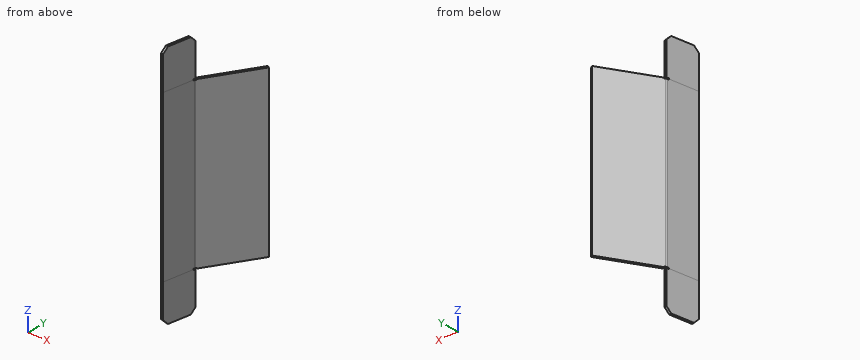
```python
from build123d import *

# Parameters (mm, degrees)
BOSS_EXTRUDE1_DEPTH      = 109.5375
BOSS_EXTRUDE1_DEPTH_BACK = 109.5375
SKETCH2_W                = 50.8
SKETCH2_H                = 42.97785953
BOSS_EXTRUDE2_DEPTH      = 3.175
CHAMFER1_SIZE            = 6.35
CONVERT_SOLID1_START     = -110.33125
CONVERT_SOLID1_DEPTH     = 220.6625
CONVERT_SOLID1_2_DEPTH   = 1.5875
CONVERT_SOLID1_START_2   = 108.74375
CONVERT_SOLID1_3_DEPTH   = 1.5875
CONVERT_SOLID1_START_3   = -108.74375
CONVERT_SOLID1_4_DEPTH   = 217.4875


# Read off the part's stored shape, not the designer's step: Convert-Solid1
with BuildPart() as part:
    # Sketch1 → Boss-Extrude1 (new, two sides: drawn at the far end of the back side and taken through both)
    with BuildSketch(Plane.XY.offset(-BOSS_EXTRUDE1_DEPTH_BACK)):
        Polygon((640.29736406, 709.2417051), (646.924037824, 751.080876614), (687.413907929, 818.467336674), (684.69240175, 820.102582562), (643.884672043, 752.187115289), (637.161453578, 709.738384527), align=None)
    extrude(amount=BOSS_EXTRUDE1_DEPTH + BOSS_EXTRUDE1_DEPTH_BACK)

    # Sketch2 → Boss-Extrude2 (add)
    with BuildSketch(Plane(origin=(511.908391779, -81.078324129, 0), x_dir=(0, 0, 1), z_dir=(-0.9876883405951397, 0.1564344650402187, 0))):
        with Locations((-134.9375, 822.16326817)):
            Rectangle(SKETCH2_W, SKETCH2_H)
        with Locations((134.9375, 822.16326817)):
            Rectangle(SKETCH2_W, SKETCH2_H)
    extrude(amount=-BOSS_EXTRUDE2_DEPTH)

    # Chamfer1
    chamfer1_edges = [part.edges().sort_by_distance(p)[0] for p in [
        (645.452627283, 751.938775576, -160.3375),
        (638.729408819, 709.490044814, -160.3375),
        (645.452627283, 751.938775576, 160.3375),
        (638.729408819, 709.490044814, 160.3375),
    ]]
    chamfer(chamfer1_edges, length=CHAMFER1_SIZE)

    # Convert-Solid1 outline → Convert-Solid1 (cut)
    with BuildSketch(Plane.XY.offset(CONVERT_SOLID1_START)):
        with BuildLine():
            Line((644.520391245, 753.245129714), (643.884672043, 752.187115289))
            Line((643.884672043, 752.187115289), (643.691582642, 750.967996791))
            ThreePointArc((643.691582642, 750.967996791), (643.996355462, 752.146465849), (644.520391245, 753.245129714))
        make_face()
    extrude(amount=CONVERT_SOLID1_DEPTH, mode=Mode.SUBTRACT)

    # Convert-Solid1 2 outline → Convert-Solid1 2 (cut)
    with BuildSketch(Plane.XY.offset(CONVERT_SOLID1_START)):
        with BuildLine():
            Line((647.241897425, 751.609883826), (648.059520369, 752.970636916))
            Line((648.059520369, 752.970636916), (645.338014189, 754.605882804))
            Line((645.338014189, 754.605882804), (644.520391245, 753.245129714))
            ThreePointArc((644.520391245, 753.245129714), (643.996355462, 752.146465849), (643.691582642, 750.967996791))
            Line((643.691582642, 750.967996791), (643.408575407, 749.181159432))
            Line((643.408575407, 749.181159432), (646.544485888, 748.684480005))
            Line((646.544485888, 748.684480005), (646.924037824, 751.080876614))
            Line((646.924037824, 751.080876614), (647.241897425, 751.609883826))
        make_face()
    extrude(amount=CONVERT_SOLID1_2_DEPTH, mode=Mode.SUBTRACT)

    # Convert-Solid1 3 outline → Convert-Solid1 3 (cut)
    with BuildSketch(Plane.XY.offset(CONVERT_SOLID1_START_2)):
        with BuildLine():
            Line((647.241897425, 751.609883826), (648.059520369, 752.970636916))
            Line((648.059520369, 752.970636916), (645.338014189, 754.605882804))
            Line((645.338014189, 754.605882804), (644.520391245, 753.245129714))
            ThreePointArc((644.520391245, 753.245129714), (643.996355462, 752.146465849), (643.691582642, 750.967996791))
            Line((643.691582642, 750.967996791), (643.408575407, 749.181159432))
            Line((643.408575407, 749.181159432), (646.544485888, 748.684480005))
            Line((646.544485888, 748.684480005), (646.924037824, 751.080876614))
            Line((646.924037824, 751.080876614), (647.241897425, 751.609883826))
        make_face()
    extrude(amount=CONVERT_SOLID1_3_DEPTH, mode=Mode.SUBTRACT)

    # Convert-Solid1 4 outline → Convert-Solid1 4 (add)
    with BuildSketch(Plane.XY.offset(CONVERT_SOLID1_START_3)):
        with BuildLine():
            ThreePointArc((646.827493123, 750.471317365), (646.979879533, 751.060551894), (647.241897425, 751.609883826))
            Line((647.241897425, 751.609883826), (646.924037824, 751.080876614))
            Line((646.924037824, 751.080876614), (646.827493123, 750.471317365))
        make_face()
    extrude(amount=CONVERT_SOLID1_4_DEPTH)


solid = part.part
```
Verification items for the finished model (mm, model axes). Round coordinates to 2 decimals unless told otherwise and drop trailing zeros. Order: outer loops, then holes, each group sorted by start corner. A loop starts at its lowest first (then second) coordinate and runs counter-clockwise, first axis right, second up. Notation, with made-up numbers: (84.25, -0.75) -> (104.25, -0.75) arc R27 ccw to (104.25, 24.25) -> close; hole circle Ø10 at (33, 72). An arc over 180 degrees is marked (long way). Put each result on its own line as item: value. Start each with the question number.
(1) Section check D-D (z = 113.5). Enter the section's corners in (x, y), then the cut area to 3 significant figures.
(2) Section check C-C (x = 671). Enter the section's corners in (y, z).
(3) Material ranges on line 1 along Z through (x, y) = (666, 784.5); line 2 along Y through (x, z) = (661.5, 50); line 3 along Y through (x, z) = (653, 6.5), recorded low to high.
(4) Depth check by flat-ended pin: pin 1 Ø3 at (x, z) = (681, 95.5) entering from +Y; pin 2 Ø12 at (x, z) = (666.5, -15) entering from +Y; pin 3 Ø5 at (x, y) = (645, 752) entering from -Z. Enter the tip coordinate at first touch or a pass-through.
(5) Section check B-B (y = 725.5). Enter the section's corners in (x, z).
Completed:
1. outline: (637.16, 709.74) -> (640.3, 709.24) -> (647.02, 751.69) -> (643.88, 752.19) -> close
1. area: 136 mm2
2. outline: (791.15, -109.54) -> (797.31, -109.54) -> (797.31, 109.54) -> (791.15, 109.54) -> close
3. line 1: z = -109.54 to 109.54
3. line 2: y = 775.34 to 781.5
3. line 3: y = 761.19 to 767.36
4. pin 1: stops at y = 816.45
4. pin 2: stops at y = 799.81
4. pin 3: stops at z = -156.5
5. outline: (639.66, -160.34) -> (642.87, -160.34) -> (642.87, 160.34) -> (639.66, 160.34) -> close
